Autodesk Inventor part; units mm, degrees
ref_plane "Startebene" through (0, 0, 0) normal (0, 0, 1) x (1, 0, 0)
ref_plane "Endebene" through (0, 0, 70) normal (0, 0, 1) x (1, 0, 0)
ref_plane "YZ Plane" through (0, 0, 0) normal (1, 0, 0) x (0, 1, 0)
ref_plane "Startebene" through (0, 0, 0) normal (0, 0, 1) x (1, 0, 0)
ref_plane "Endebene" through (0, 0, 70) normal (0, 0, 1) x (1, 0, 0)
sketch "Skizze" plane through (0, 0, 0) normal (0, 0, 1) x (1, 0, 0)
  arc A0 (-4.5287, -3.2559) -> (-3.65, -1.1346) centre (-6.65, -1.1346) ccw
  line L0 (-3.65, -1.1346) -> (-3.65, 1.1346)
  circle A1 centre (0, 0) radius 2.15
  line L1 (1.1346, -3.65) -> (-1.1346, -3.65)
  arc A2 (-1.1346, -3.65) -> (-3.2559, -4.5287) centre (-1.1346, -6.65) ccw
  line L2 (-6.779, -5.5062) -> (-4.5287, -3.2559)
  line L3 (-3.2559, -4.5287) -> (-5.5062, -6.779)
  arc A3 (-2.5, -8.5) -> (-2.8, -8.2) centre (-2.8, -8.5) ccw
  line L4 (-2.5, -8.5) -> (-2.5, -9.2)
  line L5 (-4.9176, -8.2) -> (-2.8, -8.2)
  arc A4 (-5.5062, -6.779) -> (-4.9176, -8.2) centre (-4.9176, -7.3676) ccw
  arc A5 (-3.3, -10) -> (-2.5, -9.2) centre (-3.3, -9.2) ccw
  line L6 (-3.3, -10) -> (-8, -10)
  line L7 (10, -3.3) -> (10, -8)
  line L8 (5.5062, -6.779) -> (3.2559, -4.5287)
  arc A6 (6.779, -5.5062) -> (8.2, -4.9176) centre (7.3676, -4.9176) ccw
  arc A7 (3.2559, -4.5287) -> (1.1346, -3.65) centre (1.1346, -6.65) ccw
  line L9 (4.5287, -3.2559) -> (6.779, -5.5062)
  arc A8 (3.65, -1.1346) -> (4.5287, -3.2559) centre (6.65, -1.1346) ccw
  arc A9 (8.5, -2.5) -> (8.2, -2.8) centre (8.5, -2.8) ccw
  line L10 (3.65, 1.1346) -> (3.65, -1.1346)
  line L11 (8.5, -2.5) -> (9.2, -2.5)
  arc A10 (10, -3.3) -> (9.2, -2.5) centre (9.2, -3.3) ccw
  line L12 (8.2, -4.9176) -> (8.2, -2.8)
  line L13 (2.5, 8.5) -> (2.5, 9.2)
  arc A11 (2.5, 8.5) -> (2.8, 8.2) centre (2.8, 8.5) ccw
  arc A12 (1.1346, 3.65) -> (3.2559, 4.5287) centre (1.1346, 6.65) ccw
  line L14 (-1.1346, 3.65) -> (1.1346, 3.65)
  arc A13 (3.3, 10) -> (2.5, 9.2) centre (3.3, 9.2) ccw
  line L15 (4.9176, 8.2) -> (2.8, 8.2)
  arc A14 (4.5287, 3.2559) -> (3.65, 1.1346) centre (6.65, 1.1346) ccw
  line L16 (3.2559, 4.5287) -> (5.5062, 6.779)
  arc A15 (5.5062, 6.779) -> (4.9176, 8.2) centre (4.9176, 7.3676) ccw
  line L17 (6.779, 5.5062) -> (4.5287, 3.2559)
  line L18 (3.3, 10) -> (8, 10)
  arc A16 (10, 8) -> (8, 10) centre (8, 8) ccw
  line L19 (8.2, 2.8) -> (8.2, 4.9176)
  line L20 (10, 8) -> (10, 3.3)
  arc A17 (8.2, 4.9176) -> (6.779, 5.5062) centre (7.3676, 4.9176) ccw
  line L21 (-2.8, 8.2) -> (-4.9176, 8.2)
  line L22 (-2.5, 9.2) -> (-2.5, 8.5)
  arc A18 (-2.5, 9.2) -> (-3.3, 10) centre (-3.3, 9.2) ccw
  arc A19 (-2.8, 8.2) -> (-2.5, 8.5) centre (-2.8, 8.5) ccw
  arc A20 (-3.65, 1.1346) -> (-4.5287, 3.2559) centre (-6.65, 1.1346) ccw
  arc A21 (-3.2559, 4.5287) -> (-1.1346, 3.65) centre (-1.1346, 6.65) ccw
  arc A22 (4.9176, -8.2) -> (5.5062, -6.779) centre (4.9176, -7.3676) ccw
  arc A23 (8, -10) -> (10, -8) centre (8, -8) ccw
  line L23 (2.8, -8.2) -> (4.9176, -8.2)
  line L24 (8, -10) -> (3.3, -10)
  arc A24 (2.8, -8.2) -> (2.5, -8.5) centre (2.8, -8.5) ccw
  arc A25 (2.5, -9.2) -> (3.3, -10) centre (3.3, -9.2) ccw
  line L25 (2.5, -9.2) -> (2.5, -8.5)
  arc A26 (8.2, 2.8) -> (8.5, 2.5) centre (8.5, 2.8) ccw
  line L26 (9.2, 2.5) -> (8.5, 2.5)
  arc A27 (9.2, 2.5) -> (10, 3.3) centre (9.2, 3.3) ccw
  arc A28 (-4.9176, 8.2) -> (-5.5062, 6.779) centre (-4.9176, 7.3676) ccw
  line L27 (-8, 10) -> (-3.3, 10)
  line L28 (-5.5062, 6.779) -> (-3.2559, 4.5287)
  arc A29 (-8, 10) -> (-10, 8) centre (-8, 8) ccw
  arc A30 (-6.779, 5.5062) -> (-8.2, 4.9176) centre (-7.3676, 4.9176) ccw
  line L29 (-10, 3.3) -> (-10, 8)
  line L30 (-8.2, 4.9176) -> (-8.2, 2.8)
  arc A31 (-8.5, 2.5) -> (-8.2, 2.8) centre (-8.5, 2.8) ccw
  line L31 (-8.5, 2.5) -> (-9.2, 2.5)
  arc A32 (-10, 3.3) -> (-9.2, 2.5) centre (-9.2, 3.3) ccw
  line L32 (-4.5287, 3.2559) -> (-6.779, 5.5062)
  line L33 (-10, -8) -> (-10, -3.3)
  arc A33 (-8.2, -4.9176) -> (-6.779, -5.5062) centre (-7.3676, -4.9176) ccw
  arc A34 (-10, -8) -> (-8, -10) centre (-8, -8) ccw
  line L34 (-10, -8) -> (-10, -3.3)
  arc A35 (-8.2, -2.8) -> (-8.5, -2.5) centre (-8.5, -2.8) ccw
  line L35 (-9.2, -2.5) -> (-8.5, -2.5)
  arc A36 (-9.2, -2.5) -> (-10, -3.3) centre (-9.2, -3.3) ccw
  line L36 (-8.2, -2.8) -> (-8.2, -4.9176)
  dimension "d4" = 4.3
  dimension "d5" = 6.35
  dimension "d6" = 10
  dimension "d7" = 2.5
  dimension "d8" = 5.8
  dimension "d9" = 10.5
  dimension "d10" = 3
  dimension "d11" = 7.5
  dimension "d12" = 12.5
  dimension "d13" = 13.65
  dimension "d14" = 5.7
  dimension "d15" = 10.7
  dimension "d16" = 1.15
  dimension "d17" = 6.15
  dimension "d18" = 1.8
  dimension "d19" = 0.8
  dimension "d20" = 0.3
  dimension "d21" = 2
  dimension "d22" = 0.8324
  dimension "d23" = 45
  dimension "d24" = 90
  dimension "d25" = 90
  dimension "d26" = 1.8
  dimension "d27" = 18.2
  dimension "d28" = 20
  dimension "d29" = 5
  dimension "d30" = 7.5
  dimension "d31" = 1.8
  dimension "d32" = 0.9
  dimension "d33" = 0.9
  dimension "d34" = 20
extrude "Körper" add sketch "Skizze" along normal up to surface (70 mm away) from surface at 0
sketch "Skizze6" plane through (0, 0, 0) normal (0, 0, 1) x (1, 0, 0)
  line L0 (0, 0) -> (10, 0)
ref_plane "Arbeitsebene4" through (0, 0, 0) normal (0, -1, 0) x (1, 0, 0)
sketch "Skizze7" plane through (0, 0, 0) normal (0, -1, 0) x (1, 0, 0)
  line L0 (-2, 0) -> (12, 0)
  line L1 (-2, 70) -> (12, 70)
  dimension "d43" = 70
equation "\"G_OFFSET_START\" = 0"
equation "\"G_OFFSET_END\" = 0"
equation "\"G_L\" = d43"
Check sheet for the modelled part. Datum: model origin and axes. Units: mm. A direction names the side the tool comes from. Round coordinates to 2 decimals unless told otherwise and drop trailing zeros. Order: outer loops, then holes, each group sorted by start corner. A loop starts at its lowest first (then second) coordinate and runs counter-clockwise, first axis right, second up. Notation, with made-up numbers: M 26.5,7.25 L 34.5,7.25 A27 cw 34.5,39.25 Z; hole C 28,-15 d11. An arc over 180 degrees is marked long. Answer in a Markdown table with one row per item.
(1) Gauge pin test, flat ends, axial feed: pin 1 (1 mm diameter, centred on y = 0, z = 40, fed in from -X); pin 2 (0.8 mm diameter, centred on y = -9, z = 24, fed in from -X); pin 3 (0.6 mm diameter, centred on y = 8.5, z = 48.5, fed in from +X). Record the tip position at first contact, or that the pin passes through.
Findings:
| item | result |
|---|---|
| pin 1 | stops at x = -3.65 |
| pin 2 | stops at x = -9.91 |
| pin 3 | stops at x = 9.99 |
(2) Section check A-A on x = 0. Record the boundary of the cut face in (y, z).
Findings:
| item | result |
|---|---|
| outline | M -3.65,0 L -2.15,0 L -2.15,70 L -3.65,70 Z; M 2.15,0 L 3.65,0 L 3.65,70 L 2.15,70 Z |
(3) Material ranges on line 1 along Y through (x, z) = (0, 20); line 2 along X through (y, z) = (-4.25, 28.5); line 3 along Y through (x, z) = (-3, 28), recorded low to high. Write a range as from..to.
Findings:
| item | result |
|---|---|
| line 1 | y = -3.65..-2.15, 2.15..3.65 |
| line 2 | x = -10..-8.2, -5.52..-2.93, 2.93..5.52, 8.2..10 |
| line 3 | y = -9.94..-8.2, -4.3..4.3, 8.2..9.94 |
(4) Set-up check for faces 1 (the flat face through (-6, -10, 35)), 2 (the flat face through (-5.64, 4.37, 34.51)): record each of +Z, -Z, +X, -X, +Y, -Y from which the full face is reachable in a straight line by a thin tool's end or side.
Findings:
| item | result |
|---|---|
| face 1 | +Z, -Z, +X, -X, -Y |
| face 2 | +Z, -Z |
(5) Draft check along X on faces 3 (the flat face through (-4.37, -5.64, 34.51)), 4 (the cylindrical face through (7.673, 5.692, 34.51)), 5 (the flat face through (-0.1, 2.4, 70)), 6 (the flat face through (-10, -6, 35)). Enter one of: +X half, -X half, draft (parallel to the pull), parting line (faces both ways), or undercut.
Findings:
| item | result |
|---|---|
| face 3 | undercut |
| face 4 | undercut |
| face 5 | draft |
| face 6 | -X half |
